from build123d import *

# Parameters (mm, degrees)
F3_W     = 173.5
F3_H     = 117.6
F4_DEPTH = 15
F2_W     = 155.5
F2_H     = 97.6
F5_DEPTH = 15
F1_W     = 161.5
F1_H     = 105.6
F6_DEPTH = 13


with BuildPart() as f4:
    # F3 (on face) → F4 (new body)
    with BuildSketch(Plane.XY):
        Rectangle(F3_W, F3_H)
    extrude(amount=F4_DEPTH)

    # F2 (on face) → F5 (cut)
    with BuildSketch(Plane.XY):
        with Locations((1, 2.5)):
            Rectangle(F2_W, F2_H)
    extrude(amount=F5_DEPTH, mode=Mode.SUBTRACT)

    # F1 (on Top) → F6 (cut)
    with BuildSketch(Plane.XY):
        Rectangle(F1_W, F1_H)
    extrude(amount=-F6_DEPTH, mode=Mode.SUBTRACT)


solid = f4.part
Geometry: final body of the model. Coordinates: model frame, mm. A direction names the side the tool comes from. Coordinates: 2 decimals unless noted, no trailing zeros. Loops run counter-clockwise (first coordinate to the right, second up) from the corner with the lowest first, then second, coordinate; pieces in that order, holes last. Notation, with made-up numbers: M 8.25,25 L 13.25,25 A11 cw 13.25,29 Z; hole C -18,-12 d7. An arc over 180 degrees is marked long. One line per item, written item: value. Start each with the question number.
1) Material intervals for L1, parallel to X at y = 7, z = 12; L2, parallel to Y at x = 10, z = 12.75, sorted ascending. Write a range as from..to.
2) Cut plane C-C (z = 5.25). Return loops of the section in (x, y).
3) Cut plane B-B (y = -29.5). Return loops of the section in (x, z), then the cut area to 3 significant figures.
4) Cut plane A-A (x = 60). Return loops of the section in (y, z).
5) Draft query along Y for faces 3 (the flat face through (0, 51.3, 7)), 4 (the flat face through (-1, -58.8, 7)), 5 (the flat face through (-13, -48, 0)), 6 (the flat face through (-1, 58.8, 7)). Return one class per face: released by +Y, released by -Y, zero draft, split by the parting line, or undercut.
6) Reachability of faces 1 (the flat face through (86.75, -1, 7)), 2 (the flat face through (0, -46.3, 7)) from +Z, -Z, +X, -X, +Y, -Y: full face, straight path, thin tool, end or side. Return the list, or none.
Evaluation:
1. L1: -86.75..-76.75, 78.75..86.75
1. L2: -58.8..-46.3, 51.3..58.8
2. outline: M -86.75,-58.8 L 86.75,-58.8 L 86.75,58.8 L -86.75,58.8 Z; hole M -76.75,-46.3 L 78.75,-46.3 L 78.75,51.3 L -76.75,51.3 Z
3. outline: M -86.75,0 L -76.75,0 L -76.75,15 L -86.75,15 Z; M 78.75,0 L 86.75,0 L 86.75,15 L 78.75,15 Z
3. area: 270 mm^2
4. outline: M -58.8,0 L -46.3,0 L -46.3,15 L -58.8,15 Z; M 51.3,0 L 58.8,0 L 58.8,15 L 51.3,15 Z
5. face 3: undercut
5. face 4: released by -Y
5. face 5: zero draft
5. face 6: released by +Y
6. face 1: +Z, -Z, +X, +Y, -Y
6. face 2: +Z, -Z
